Verification items for the finished model (mm, model axes). A direction names the side the tool comes from. Round coordinates to 2 decimals unless told otherwise and drop trailing zeros. Order: outer loops, then holes, each group sorted by start corner. A loop starts at its lowest first (then second) coordinate and runs counter-clockwise, first axis right, second up. Notation, with made-up numbers: (43.25, 33.5) -> (53.25, 33.5) arc R17 cw to (53.25, 56.5) -> close; hole circle Ø1 at (25.25, 33). An arc over 180 degrees is marked (long way). Write item = value, one per line. Start each with the question number.
from build123d import *

# Parameters (mm, degrees)
BOSS_EXTRUDE3_DEPTH = 15
BOSS_EXTRUDE6_DEPTH = 63
SKETCH8_R           = 10
CUT_EXTRUDE1_DEPTH  = 60
BOSS_EXTRUDE8_DEPTH = 10


with BuildPart() as part:
    # Sketch4 → Boss-Extrude3 (new body)
    with BuildSketch(Plane(origin=(0, 0, 0), x_dir=(0, 0, -1), z_dir=(1, 0, 0))):
        Polygon((0, 0), (0, 62.333333333), (-87.595238095, 62.333333333), (-87.595238095, 45), (-22.595238095, 45), (-22.595238095, 15), (-87.595238095, 15), (-87.595238095, 0), align=None)
    extrude(amount=BOSS_EXTRUDE3_DEPTH)

    # Sketch7 → Boss-Extrude6 (add)
    with BuildSketch(Plane(origin=(0, 62.333333333, 0), x_dir=(1, 0, 0), z_dir=(0, 1, 0))):
        with BuildLine():
            Line((15, 0), (15, 70.864702181))
            ThreePointArc((15, 70.864702181), (-15.798204654, 101.662906835), (-46.596409308, 70.864702181))
            Line((-46.596409308, 70.864702181), (-46.596409308, 0))
            Line((-46.596409308, 0), (0, 0))
            Line((0, 0), (15, 0))
        make_face()
    extrude(amount=-BOSS_EXTRUDE6_DEPTH)

    # Sketch8 → Cut-Extrude1 (cut)
    with BuildSketch(Plane(origin=(0, 62.333333333, 0), x_dir=(1, 0, 0), z_dir=(0, 1, 0))):
        with Locations(Location((-15.914385608, 80.072094145, 0), (0, 0, 270))):
            Circle(SKETCH8_R)
    extrude(amount=-CUT_EXTRUDE1_DEPTH, mode=Mode.SUBTRACT)

    # Sketch12 → Boss-Extrude8 (add)
    with BuildSketch(Plane(origin=(0, 20, 0), x_dir=(1, 0, 0), z_dir=(0, 1, 0))):
        Polygon((-46.596409308, 0), (0, 0), (0, -22.515812616), align=None)
    extrude(amount=BOSS_EXTRUDE8_DEPTH)


solid = part.part
(1) Depth check by flat-ended pin: pin 1 (4.5 mm diameter, centred on x = 6, z = 56, fed in from -Y); pin 2 (10 mm diameter, centred on x = -19, z = -80, fed in from +Y); pin 3 (6 mm diameter, centred on x = -27.5, y = 4.5, fed in from +Z); pin 4 (7 mm diameter, centred on x = -31, z = 13.5, fed in from -Y). Enter the tip coordinate at first touch or a pass-through.
(2) Cross-section at C-C (x = -43). Enter the section's corners in (y, z).
(3) Cross-section at D-D (z = 18.5). Enter the section's corners in (x, y).
(4) Scan lines: line 1 along Z through (x, y) = (-15, 11); line 2 along X through (y, z) = (5, 31.5); line 3 along Z through (x, y) = (-13, 58.5). Record each from-to range of solid material in increasing order. Write a range as from..to.
(5) Cross-section at B-B (y = 10). Enter the section's corners in (x, z).
(6) Draft check along Y on faces 5 (the flat face through (7, 45, 56)), 6 (the flat face through (7, 30, 22.595)), 7 (the flat face through (7, 0, 44)), 8 (the flat face through (15, 31, -8)). Enter one of: +Y half, -Y half, draft (parallel to the pull), parting line (faces both ways), or undercut.
(7) Set-up check for faces 1 (the flat face through (-18, 20, 9)), 2 (the flat face through (7, 15, 55)), 3 (the flat face through (-16, 2.333, -80)), 4 (the flat face through (-24, 46, 0)): record each of +Z, -Z, +X, -X, +Y, -Y from which the full face is reachable in a straight line by a thin tool's end or side.
(8) Cross-section at A-A (z = 64). Enter the section's corners in (x, y), and give its area (3 significant figures).
Outcome:
q1.pin_1 = 0
q1.pin_2 = 2.33
q1.pin_3 = 0
q1.pin_4 = through
q2.outline = (-0.67, -85.31) -> (62.33, -85.31) -> (62.33, 0) -> (30, 0) -> (30, 1.74) -> (20, 1.74) -> (20, 0) -> (-0.67, 0) -> close
q3.outline = (-8.31, 20) -> (0, 20) -> (0, 0) -> (15, 0) -> (15, 62.33) -> (0, 62.33) -> (0, 30) -> (-8.31, 30) -> close
q4.line_1 = -101.65..-90.03, -70.11..0
q4.line_2 = 0..15
q4.line_3 = -101.54..-89.64, -70.51..0
q5.outline = (-46.6, -70.86) arc R30.8 ccw to (15, -70.86) -> (15, 87.6) -> (0, 87.6) -> (0, 0) -> (-46.6, 0) -> close; hole circle Ø20 at (-15.91, -80.07)
q6.face_5 = undercut
q6.face_6 = undercut
q6.face_7 = -Y half
q6.face_8 = draft
q7.face_1 = +Z, -X, -Y
q7.face_2 = +Z, +X, -X
q7.face_3 = +Y
q7.face_4 = +Z, -X, +Y
q8.outline = (0, 0) -> (15, 0) -> (15, 15) -> (0, 15) -> close; (0, 45) -> (15, 45) -> (15, 62.33) -> (0, 62.33) -> close
q8.area = 485 mm^2
